from build123d import *

# Parameters (mm, degrees)
SKETCH1_R           = 6.223
SKETCH1_R_2         = 3.175
BOSS_EXTRUDE1_DEPTH = 2.54
SKETCH1_3_R         = 4.233333333
BOSS_EXTRUDE2_DEPTH = 12.7
SKETCH2_R           = 8.89
SKETCH2_R_2         = 6.223
CUT_EXTRUDE2_DEPTH  = 0.508


with BuildPart() as part:
    # Sketch1 → Boss-Extrude1 (new body)
    with BuildSketch(Plane(origin=(0, 0, 0), x_dir=(1, 0, 0), z_dir=(0, 1, 0))):
        with BuildLine():
            Line((-27.479757553, 19.069204536), (-27.479757553, -19.069204536))
            add(Edge.make_bspline(
                [(-106.608177043, 0), (-106.607181853, -0.336221439), (-106.553109217, -1.172470844), (-106.231145111, -2.643099261), (-105.439203383, -4.475217401), (-104.022724766, -6.504348411), (-101.933239026, -8.571651325), (-99.191911488, -10.567556696), (-95.844996836, -12.426747292), (-91.942526077, -14.111441704), (-87.531895483, -15.599318155), (-82.657100659, -16.877133316), (-77.359343302, -17.937435613), (-71.677800746, -18.776740565), (-65.650341253, -19.395460579), (-59.313785065, -19.796574023), (-52.704246728, -19.986276309), (-45.857195612, -19.97286583), (-38.807557342, -19.767322463), (-32.659211886, -19.439565325), (-28.865800162, -19.174037811), (-27.479757553, -19.069204536)],
                knots=[0.5, 0.5, 0.5, 0.5, 0.502166769, 0.505390167, 0.509655974, 0.514947682, 0.521244711, 0.528520886, 0.536744945, 0.54588136, 0.555890751, 0.566730119, 0.57835299, 0.590709588, 0.603747039, 0.617409572, 0.631638768, 0.646373793, 0.661551658, 0.677107483, 0.686069724, 0.686069724, 0.686069724, 0.686069724], degree=3))
            add(Edge.make_bspline(
                [(-106.608177043, 0), (-106.607181853, 0.336221439), (-106.553109217, 1.172470844), (-106.231145111, 2.643099261), (-105.439203383, 4.475217401), (-104.022724766, 6.504348411), (-101.933239026, 8.571651325), (-99.191911488, 10.567556696), (-95.844996836, 12.426747292), (-92.90409582, 13.696332592), (-91.099565345, 14.363844596), (-90.622228407, 14.533411548)],
                knots=[0.5, 0.5, 0.5, 0.5, 0.502166769, 0.505390167, 0.509655974, 0.514947682, 0.521244711, 0.528520886, 0.536744945, 0.54588136, 0.54914681, 0.54914681, 0.54914681, 0.54914681], degree=3))
            add(Edge.make_bspline(
                [(-90.622228407, 14.533411548), (-78.676623194, 33.624035256), (-75.814032891, 56.696401983), (-76.556217491, 62.136682092)],
                knots=[0, 0, 0, 0, 1, 1, 1, 1], degree=3))
            ThreePointArc((-76.556217491, 62.136682092), (-72.773341431, 68.985549888), (-66.748032241, 63.994278454))
            add(Edge.make_bspline(
                [(-66.748032241, 63.994278454), (-59.662783709, 42.677267871), (-27.479757553, 19.069204536)],
                knots=[0, 0, 0, 1, 1, 1], degree=2))
        make_face()
        with Locations(Location((-71.828032241, 0, 0), (0, 0, 270))):
            Circle(SKETCH1_R, mode=Mode.SUBTRACT)
        with Locations(Location((-71.828032241, 63.994278454, 0), (0, 0, 90))):
            Circle(SKETCH1_R_2, mode=Mode.SUBTRACT)
    extrude(amount=BOSS_EXTRUDE1_DEPTH)

    # Sketch1_3 → Boss-Extrude2 (add)
    with BuildSketch(Plane(origin=(0, 0, 0), x_dir=(1, 0, 0), z_dir=(0, 1, 0))):
        with BuildLine():
            Line((-42.848770143, -14.977337356), (-27.479757553, -13.544433585))
            Line((-27.479757553, -13.544433585), (-27.479757553, 13.544433585))
            Line((-27.479757553, 13.544433585), (-42.848770143, 14.977337356))
            Line((-42.848770143, 14.977337356), (-45.666032241, 15.24))
            ThreePointArc((-45.666032241, 15.24), (-60.906032241, 0), (-45.666032241, -15.24))
            Line((-45.666032241, -15.24), (-42.848770143, -14.977337356))
        make_face()
        with Locations(Location((-93.062306932, 0, 0), (0, 0, 270))):
            Circle(SKETCH1_3_R)
    extrude(amount=-BOSS_EXTRUDE2_DEPTH)

    # Sketch2 → Cut-Extrude2 (cut)
    with BuildSketch(Plane(origin=(0, 2.54, 0), x_dir=(1, 0, 0), z_dir=(0, 1, 0))):
        with Locations(Location((-71.828032241, 0, 0), (0, 0, 270))):
            Circle(SKETCH2_R)
        with Locations(Location((-71.828032241, 0, 0), (0, 0, 270))):
            Circle(SKETCH2_R_2, mode=Mode.SUBTRACT)
    extrude(amount=-CUT_EXTRUDE2_DEPTH, mode=Mode.SUBTRACT)


solid = part.part
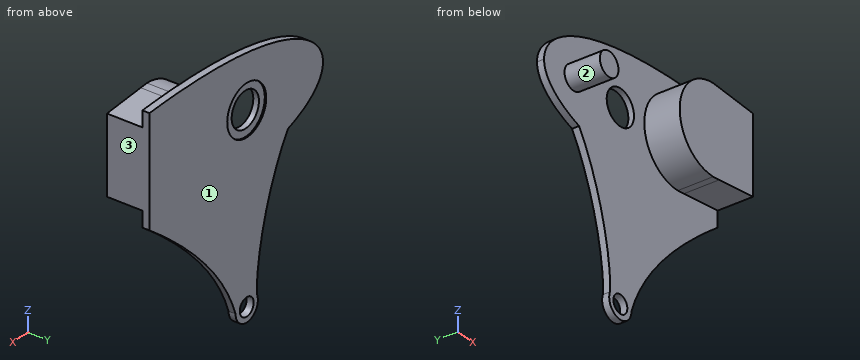
Source: CAD feature listing. Evaluate the final solid. Frame: model axes, mm. Face numbers are marked on the shaded views. Round coordinates to 2 decimals unless told otherwise and drop trailing zeros. Loops run counter-clockwise (first coordinate to the right, second up) from the corner with the lowest first, then second, coordinate; pieces in that order, holes last. Notation, with made-up numbers: (63, -30) - (100, -30) arc R13 ccw to (100, -24) - close; hole circle Ø5 at (43, 41). An arc over 180 degrees is marked (long way). Write item = value, one per line. Start each with the question number.
Item 1: Section query A-A on y = -5.25. Output: boundary loops of the cut face in (x, z).
Item 2: Mould query, pull axis X, two halves, no side actions, for the marked faces 1, 2 and 3. Classes: released by +X, released by -X, zero draft, split by the parting line, or undercut.
Item 3: Material intervals for line 1 (X direction, y = 2.2, z = 0); line 2 (Y direction, x = -79.5, z = -20); line 3 (Z direction, x = -91, y = 1), sorted ascending.
Item 4: First-contact query: pin 1 Ø1.5 at (x, y) = (-48.5, -0.5) entering from -Z; pin 2 Ø7.5 at (x, z) = (-71.83, 0) entering from -Y; pin 3 Ø9 at (x, z) = (-74.5, -1.5) entering from +Y; pin 4 Ø20.5 at (x, z) = (-71.83, 0) entering from +Y. Flat tips, straight axial feed; report the tip coordinate or a pass-through.
Results list:
q1.outline = circle Ø8.47 at (-93.06, 0); (-45.67, -15.24) - (-27.48, -13.54) - (-27.48, 13.54) - (-45.67, 15.24) arc R15.24 ccw to start
q2.face_1 = zero draft
q2.face_2 = undercut
q2.face_3 = released by +X
q3.line_1 = -106.61 to -80.72, -62.94 to -27.48
q3.line_2 = 0 to 2.54
q3.line_3 = -14.4 to 14.4
q4.pin_1 = -37.43
q4.pin_2 = through
q4.pin_3 = 2.03
q4.pin_4 = 2.54
